For this review, take the finished solid that the model builds, in its own axes (mm). A direction names the side the tool comes from. Coordinates: 2 decimals unless noted, no trailing zeros. Loops run counter-clockwise (first coordinate to the right, second up) from the corner with the lowest first, then second, coordinate; pieces in that order, holes last. Notation, with made-up numbers: M 24,24 L 65,24 A30 ccw 65,61 Z; hole C -7,15.5 d3. An arc over 180 degrees is marked long. Put each result on its own line as item: value.
```python
from build123d import *

# Parameters (mm, degrees)
SKETCH_R          = 10.5
SKETCH_R_2        = 1.46
PAD_DEPTH         = 21.34
FILLET_R          = 0.5
SKETCH001_R       = 0.45
PAD001_DEPTH      = 10.67
PAD001_DEPTH_BACK = 3.5


with BuildPart() as fillet_body:
    # Sketch → Pad (new body)
    with BuildSketch(Plane.XY.offset(0.1)):
        with Locations((7.62, 0)):
            Circle(SKETCH_R)
        with Locations((7.62, 0)):
            Circle(SKETCH_R_2, mode=Mode.SUBTRACT)
    extrude(amount=PAD_DEPTH)

    # Fillet
    fillet_edges = [fillet_body.edges().sort_by_distance(p)[0] for p in [
        (6.16, 0, 21.44),
        (-2.88, 0, 21.44),
        (-2.88, 0, 0.1),
    ]]
    fillet(fillet_edges, radius=FILLET_R)


with BuildPart() as obj1:
    # Sketch001 → Pad001 (new body, two sides)
    with BuildSketch(Plane.XY.offset(0.5)) as pad001_sk:
        Circle(SKETCH001_R)
        with Locations((15.24, 0)):
            Circle(SKETCH001_R)
    extrude(amount=PAD001_DEPTH)
    extrude(pad001_sk.sketch, amount=-PAD001_DEPTH_BACK)

    # obj1: union Fillet body
    add(fillet_body.part)


solid = obj1.part
```
(1) Draft analysis for pull direction X (two halves, no side actions). For faces 1 (the cylindrical face through (14.79, 0.02, -1.43)), 2 (the flat face through (15, 0, -3)), 3 (the cylindrical face through (-0.119, 7.096, 10.628)), state which applies: +X half, -X half, draft (parallel to the pull), parting line (faces both ways), or undercut.
Determined:
face 1: undercut
face 2: draft
face 3: parting line
(2) Add section C-C (z = 2). Write out the cut boundary in (x, y).
Determined:
outline: C 7.62,0 d21; hole C 7.62,0 d2.92
(3) Tool access review of faces 4 (the cylindrical face through (0.429, 0.135, -1.428)), 5 (the cylindrical face through (6.16, 0.06, 10.37)): name each direction out of +Z, -Z, +X, -X, +Y, -Y from which nothing blocks a thin tool from reaching the whole face with its end or side.
Determined:
face 4: -Z
face 5: +Z, -Z
(4) For pin 1 (8 mm diameter, centred on y = -7.5, z = 1, fed in from +X); pin 2 (4 mm diameter, centred on x = 4, z = 3, fed in from +Y); pin 3 (3 mm diameter, centred on x = 11.5, z = 8, fed in from -Y), all flat-tipped, find the tip position at first contact; note any pin that passes through.
Determined:
pin 1: stops at x = 17.52
pin 2: stops at y = 10.37
pin 3: stops at y = -10.23
(5) Add section B-B (y = 0). Write out the cut boundary in (x, z), plus the area to 3 significant figures.
Determined:
outline: M -2.88,0.6 A0.5 ccw -2.38,0.1 L -0.45,0.1 L -0.45,-3 L 0.45,-3 L 0.45,0.1 L 6.16,0.1 L 6.16,20.94 A0.5 ccw 5.66,21.44 L -2.38,21.44 A0.5 ccw -2.88,20.94 Z; M 9.08,0.1 L 14.79,0.1 L 14.79,-3 L 15.69,-3 L 15.69,0.1 L 17.62,0.1 A0.5 ccw 18.12,0.6 L 18.12,20.94 A0.5 ccw 17.62,21.44 L 9.58,21.44 A0.5 ccw 9.08,20.94 Z
area: 391 mm^2
(6) Add section A-A (x = 7.62). Write out the cut boundary in (y, z), plus the area to 3 significant figures.
Determined:
outline: M -10.5,0.6 A0.5 ccw -10,0.1 L -1.46,0.1 L -1.46,20.94 A0.5 ccw -1.96,21.44 L -10,21.44 A0.5 ccw -10.5,20.94 Z; M 1.46,0.1 L 10,0.1 A0.5 ccw 10.5,0.6 L 10.5,20.94 A0.5 ccw 10,21.44 L 1.96,21.44 A0.5 ccw 1.46,20.94 Z
area: 386 mm^2
(7) Wall thickness on line 1 along Y through (x, z) = (7.62, 16.5); line 2 along Z through (x, y) = (8.5, -4.25); line 3 along Y through (x, z) = (8.5, 2.75): over which ranges is each line inside the solid? List them lowest first. Write a range as [from, to].
Determined:
line 1: y = [-10.5, -1.46], [1.46, 10.5]
line 2: z = [0.1, 21.44]
line 3: y = [-10.46, -1.16], [1.16, 10.46]
